Study the drawing (mm; zero at the part's minimum x, y, z) and answer. A direction names the side the tool comes from. Coordinates: 2 decimals unless noted, no trailing zeros. Order: outer loops, then holes, each group sorted by start corner. A loop starts at its lowest first (then second) coordinate and runs counter-clockwise, first axis right, second up.
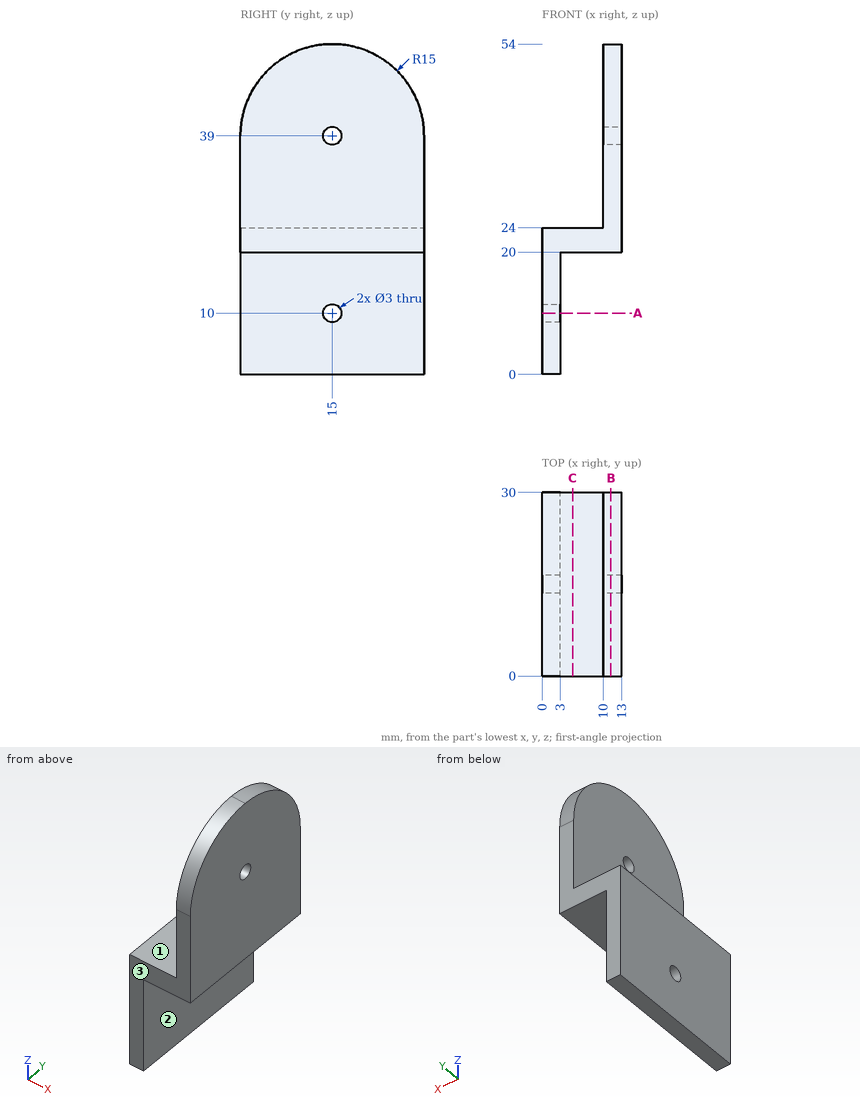
1) Straight lines are drawn through the part: line 1 (Y direction, x = 12.1, z = 39); line 2 (X direction, y = 15.5, z = 37.5); line 3 (Z direction, x = 2.5, y = 4.75). For each, find the intervals that lie inside material, in ascending order.
A:
line 1: y = 0 to 13.5, 16.5 to 30
line 2: x = 10 to 13
line 3: z = 0 to 24
2) Flat-ended cylindrical pins translate along their axes: pin 1 Ø5 at (y, z) = (15, 39) entering from -X; pin 2 Ø3 at (y, z) = (20.5, 14) entering from +X; pin 3 Ø3 at (x, y) = (8, 13.5) entering from -Z; pin 4 Ø1 at (x, y) = (3, 11) entering from -Z. Find the tip coordinate at first contact, or state that the pin passes through.
A:
pin 1: stops at x = 10
pin 2: stops at x = 3
pin 3: stops at z = 20
pin 4: stops at z = 0
3) Which of the six approach directions +Z, -Z, +X, -X, +Y, -Y give full straight-line access (tool end or side, diameter ignored) to the marked faces 1, 2 and 3?
A:
face 1: +Z, -X, +Y, -Y
face 2: -Z, +X, +Y, -Y
face 3: +Z, -Z, +X, -X, -Y
4) A cutting plane is placed at C-C, the plane x = 5. Determine the outline of the cut face in (y, z).
A:
outline: (0, 20) - (30, 20) - (30, 24) - (0, 24) - close
5) A cutting plane is placed at A-A, the plane z = 10. Determine the outline of the cut face in (x, y).
A:
outline: (0, 0) - (3, 0) - (3, 13.5) - (0, 13.5) - close; (0, 16.5) - (3, 16.5) - (3, 30) - (0, 30) - close
6) A cutting plane is placed at B-B, the plane x = 11.25. Determine the outline of the cut face in (y, z), and give its area (3 significant figures).
A:
outline: (0, 20) - (30, 20) - (30, 39) arc R15 ccw to (0, 39) - close; hole circle Ø3 at (15, 39)
area: 916 mm2
